Build history of the part. All positions in model axes, mm. A direction names the side the tool comes from. Give positions to 0.01 mm unless a question says otherwise; leave off trailing zeros. Order: outer loops, then holes, each group sorted by start corner. A loop starts at its lowest first (then second) coordinate and runs counter-clockwise, first axis right, second up. Notation, with made-up numbers: (71.25, 12.25) - (118.25, 12.25) arc R17 ccw to (118.25, 41.25) - close; hole circle Ø11 at (-33, -39). An arc over 180 degrees is marked (long way). Use a Markdown table: item, result. Add a question column.
(1) Which spindle directions (+Z, -Z, +X, -X, +Y, -Y) get a long thin tool onto all of the face, cutting with end or side? Do faces 1 (the face through (-1.65, 6.26, -7.44)), 2 (the face through (31.839, 44.038, -0.261)), 3 (the face through (-4, 0, 5)). Say none if no direction does.
(2) Slice it at B-B (x = 32.5). Write the cut outline in (y, z).
(3) Mould opens along X. For faces 4 (the face through (7, 12.7, 4)), 5 (the face through (38.1, 43, 4)), 6 (the face through (5.669, 6.439, -1.785)) say: +X half, -X half, draft (parallel to the pull), parting line (faces both ways), or undercut.
(4) Wall check: line 1 (Z direction, x = 0, y = 7.25); line 2 (X direction, y = 15, z = -5.5); line 3 (Z direction, x = 2, y = 20.5). Give the ranges that are in metal, low to high.
(5) Slice it at A-A (z = 0). Write the cut outline in (x, y).
(6) Flat gauge pins, fed straight in: pin 1 (5.5 mm diameter, centred on y = 34, z = 3, fed in from +X); pin 2 (1 mm diameter, centred on y = 31.5, z = 0.5, fed in from -X); pin 3 (4 mm diameter, centred on x = 18.5, y = 40.5, fed in from -Z); pin 4 (8 mm diameter, centred on x = 28, y = 32.5, fed in from +Z). Where does each tip first touch, or does it go through?
from build123d import *

# Parameters (mm, degrees)
F0_R     = 8.89
F0_R_2   = 5.9436
F3_R     = 8.89
F3_R_2   = 7.62
F4_DEPTH = 12.7
F5_R     = 8.89
F5_R_2   = 7.62
F6_DEPTH = 12.7


with BuildPart() as f2:
    # F2: sweep along a path in F1
    with BuildLine(Plane.XY) as f2_path:
        Line((0, 0), (0, 12.7))
        ThreePointArc((0, 12.7), (7.4394877579, 30.6605122421), (25.4, 38.1))
        Line((25.4, 38.1), (38.1, 38.1))
    # F0 (on Front) → F2 (sweep)
    with BuildSketch(Plane.XZ):
        Circle(F0_R)
        Circle(F0_R_2, mode=Mode.SUBTRACT)
    sweep(path=f2_path.line)

    # F3 (on face) → F4 (cut)
    with BuildSketch(Plane.XZ):
        Circle(F3_R)
        Circle(F3_R_2, mode=Mode.SUBTRACT)
    extrude(amount=-F4_DEPTH, mode=Mode.SUBTRACT)

    # F5 (on face) → F6 (cut)
    with BuildSketch(Plane.YZ.offset(38.1)):
        with Locations((38.1, 0)):
            Circle(F5_R)
        with Locations((38.1, 0)):
            Circle(F5_R_2, mode=Mode.SUBTRACT)
    extrude(amount=-F6_DEPTH, mode=Mode.SUBTRACT)


solid = f2.part
Solution:
| question | item | result |
|---|---|---|
| 1 | face 1 | -Y |
| 1 | face 2 | +X |
| 1 | face 3 | +Z, -Z, +X, -X, -Y |
| 2 | outline | circle Ø15.24 at (38.1, 0); hole circle Ø11.89 at (38.1, 0) |
| 3 | face 4 | draft |
| 3 | face 5 | +X half |
| 3 | face 6 | undercut |
| 4 | line 1 | -7.62 to -5.94, 5.94 to 7.62 |
| 4 | line 2 | -6.9 to -2.16, 2.37 to 7.13 |
| 4 | line 3 | -8.86 to -5.9, 5.9 to 8.86 |
| 5 | outline | (-8.89, 12.7) - (-7.62, 12.7) - (-7.62, 0) - (-5.94, 0) - (-5.94, 12.7) arc R31.34 cw to (25.4, 44.04) - (38.1, 44.04) - (38.1, 45.72) - (25.4, 45.72) - (25.4, 46.99) arc R34.29 ccw to start; (5.94, 0) - (7.62, 0) - (7.62, 12.7) - (8.89, 12.7) arc R16.51 cw to (25.4, 29.21) - (25.4, 30.48) - (38.1, 30.48) - (38.1, 32.16) - (25.4, 32.16) arc R19.46 ccw to (5.94, 12.7) - close |
| 6 | pin 1 | x = 38.1 |
| 6 | pin 2 | x = -3.58 |
| 6 | pin 3 | z = -8.8 |
| 6 | pin 4 | z = 8.51 |
